CAD build for the part. Positions are in the model's coordinates, mm. Round coordinates to 2 decimals unless told otherwise and drop trailing zeros. Order: outer loops, then holes, each group sorted by start corner. A loop starts at its lowest first (then second) coordinate and runs counter-clockwise, first axis right, second up. Notation, with made-up numbers: M -32.75,0 L -26.75,0 A21 cw -26.75,10 Z; hole C -25,63.5 d4. An arc over 180 degrees is marked long. Answer as CSV lines item,"result". Start each with the question number.
```python
from build123d import *

# Parameters (mm, degrees)
SKETCH_3_R          = 60.3
EXTRUDE_2_DEPTH     = 10
CUT_EXTRUDE_2_DEPTH = 11
FILLET_1_R          = 3
SKETCH_5_R          = 1.25
CUT_EXTRUDE_3_DEPTH = 11


with BuildPart() as part:
    # 草图3 → 凸台-拉伸2 (new body)
    with BuildSketch(Plane(origin=(0, 0, 0), x_dir=(1, 0, 0), z_dir=(0, 1, 0))):
        Circle(SKETCH_3_R)
    extrude(amount=EXTRUDE_2_DEPTH)

    # 草图4 → 切除-拉伸2 (cut, through all)
    with BuildSketch(Plane(origin=(0, 10, 0), x_dir=(1, 0, 0), z_dir=(0, 1, 0))):
        with BuildLine():
            Line((-51.556667852, 20), (-56.886641666, 20))
            ThreePointArc((-56.886641666, 20), (0, 60.3), (56.886641666, 20))
            Line((56.886641666, 20), (51.556667852, 20))
            ThreePointArc((51.556667852, 20), (0, 55.3), (-51.556667852, 20))
        make_face()
        with BuildLine():
            Line((-56.886641666, -20), (-51.556667852, -20))
            ThreePointArc((-51.556667852, -20), (0, -55.3), (51.556667852, -20))
            Line((51.556667852, -20), (56.886641666, -20))
            ThreePointArc((56.886641666, -20), (0, -60.3), (-56.886641666, -20))
        make_face()
    extrude(amount=-CUT_EXTRUDE_2_DEPTH, mode=Mode.SUBTRACT)

    # 圆角1
    fillet_1_edges = [part.edges().sort_by_distance(p)[0] for p in [
        (51.556667852, 5, -20),
        (-51.556667852, 5, -20),
        (-56.886641666, 5, -20),
        (56.886641666, 5, -20),
        (-51.556667852, 5, 20),
        (51.556667852, 5, 20),
        (56.886641666, 5, 20),
        (-56.886641666, 5, 20),
    ]]
    fillet(fillet_1_edges, radius=FILLET_1_R)

    # 草图5 → 切除-拉伸3 (cut, through all)
    with BuildSketch(Plane.XZ):
        with Locations((0, -52.7)):
            Circle(SKETCH_5_R)
        with Locations((-45.639538779, -26.35)):
            Circle(SKETCH_5_R)
        with Locations((-45.639538779, 26.35)):
            Circle(SKETCH_5_R)
        with Locations((0, 52.7)):
            Circle(SKETCH_5_R)
        with Locations((45.639538779, 26.35)):
            Circle(SKETCH_5_R)
        with Locations((45.639538779, -26.35)):
            Circle(SKETCH_5_R)
    extrude(amount=-CUT_EXTRUDE_3_DEPTH, mode=Mode.SUBTRACT)


solid = part.part
```
Q1. Drop flat-ended pins along their axis: P1, Ø0.9, axis at x = 54.5, y = 4.5, coming from the -Z side; P2, Ø1.5, axis at y = 3.5, z = -28.5, coming from the +X side; P3, Ø1.5, axis at x = -21, y = 4.5, coming from the -Z side. Give the stop position or say it passes through.
Q2. Mould opens along X. For faces 1 (the flat face through (-1, 0, -1)), 2 (the cylindrical face through (-56.52, 4.93, 19.4)), 3 (the cylindrical face through (44.39, 4.93, 26.4)) say: +X half, -X half, draft (parallel to the pull), parting line (faces both ways), or undercut.
Q3. Band-saw the part on B-B, the plane x = -39.5. Write the cut outline in (y, z), then the cut area to 3 significant figures.
Q4. Band-saw the part on A-A, the plane y = 7.5. Write the cut outline in (x, z), then the cut area to 3 significant figures.
Q5. Probe line 1 along Z through (x, y) = (-46, 7.5); line 2 along X through (y, z) = (7, 2.5); line 3 along X through (y, z) = (9, -21). List the from-to ranges inside material, lowest first. Write a range as from..to.
Q6. Band-saw the part on C-C, the plane z = 30. Write the cut outline in (x, y).
Answer:
1,P1,"stops at z = -20"
1,P2,"stops at x = 47.83"
1,P3,"stops at z = -51.46"
2,face 1,"draft"
2,face 2,"-X half"
2,face 3,"undercut"
3,outline,"M 0,-38.7 L 10,-38.7 L 10,38.7 L 0,38.7 Z"
3,area,"774 mm^2"
4,outline,"M -57.59,-17.89 A3 ccw -54.72,-20 L -53.57,-20 A3 cw -50.81,-21.82 A55.3 ccw 50.81,-21.82 A3 cw 53.57,-20 L 54.72,-20 A3 ccw 57.59,-17.89 A60.3 ccw 57.59,17.89 A3 ccw 54.72,20 L 53.57,20 A3 cw 50.81,21.82 A55.3 ccw -50.81,21.82 A3 cw -53.57,20 L -54.72,20 A3 ccw -57.59,17.89 A60.3 ccw Z; hole C -45.64,-26.35 d2.5; hole C -45.64,26.35 d2.5; hole C 0,-52.7 d2.5; hole C 0,52.7 d2.5; hole C 45.64,-26.35 d2.5; hole C 45.64,26.35 d2.5"
4,area,"9,990 mm^2"
5,line 1,"z = -30.69..-27.55, -25.15..25.15, 27.55..30.69"
5,line 2,"x = -60.25..60.25"
5,line 3,"x = -51.34..51.34"
6,outline,"M -46.46,0 L 46.46,0 L 46.46,10 L -46.46,10 Z"
